```python
from build123d import *

# Parameters (mm, degrees)
PLASTINA_DEPTH        = 5
OTVERSTIYA_DEPTH      = 86
OTVERSTIYA_DEPTH_BACK = 86
ESKIZ_OTVERSTIYA_R    = 1.65
ESKIZ_OTVERSTIYA_R_2  = 11.25


with BuildPart() as part:
    # Eskiz_kontur → Plastina (new body)
    with BuildSketch(Plane.XY):
        with BuildLine():
            Line((-60, -50), (-60, 50))
            ThreePointArc((-60, 50), (-57.071067812, 57.071067812), (-50, 60))
            Line((-50, 60), (50, 60))
            ThreePointArc((50, 60), (57.071067812, 57.071067812), (60, 50))
            Line((60, 50), (60, -50))
            ThreePointArc((60, -50), (57.071067812, -57.071067812), (50, -60))
            Line((50, -60), (-50, -60))
            ThreePointArc((-50, -60), (-57.071067812, -57.071067812), (-60, -50))
        make_face()
    extrude(amount=PLASTINA_DEPTH)

    # Eskiz_otverstiya → Otverstiya (cut, two sides: drawn at the far end of the back side and taken through both)
    with BuildSketch(Plane.XY.offset(-OTVERSTIYA_DEPTH_BACK)):
        with Locations((-50, -50)):
            Circle(ESKIZ_OTVERSTIYA_R)
        with Locations((0, -36)):
            Circle(ESKIZ_OTVERSTIYA_R)
        with Locations((-15.5, -15.5)):
            Circle(ESKIZ_OTVERSTIYA_R)
        Circle(ESKIZ_OTVERSTIYA_R_2)
        with Locations((50, -50)):
            Circle(ESKIZ_OTVERSTIYA_R)
        with Locations((15.5, -15.5)):
            Circle(ESKIZ_OTVERSTIYA_R)
        with Locations((36, 0)):
            Circle(ESKIZ_OTVERSTIYA_R)
        with Locations((-36, 0)):
            Circle(ESKIZ_OTVERSTIYA_R)
        with Locations((-15.5, 15.5)):
            Circle(ESKIZ_OTVERSTIYA_R)
        with Locations((-50, 50)):
            Circle(ESKIZ_OTVERSTIYA_R)
        with Locations((0, 36)):
            Circle(ESKIZ_OTVERSTIYA_R)
        with Locations((15.5, 15.5)):
            Circle(ESKIZ_OTVERSTIYA_R)
        with Locations((50, 50)):
            Circle(ESKIZ_OTVERSTIYA_R)
    extrude(amount=OTVERSTIYA_DEPTH + OTVERSTIYA_DEPTH_BACK, mode=Mode.SUBTRACT)


solid = part.part
```
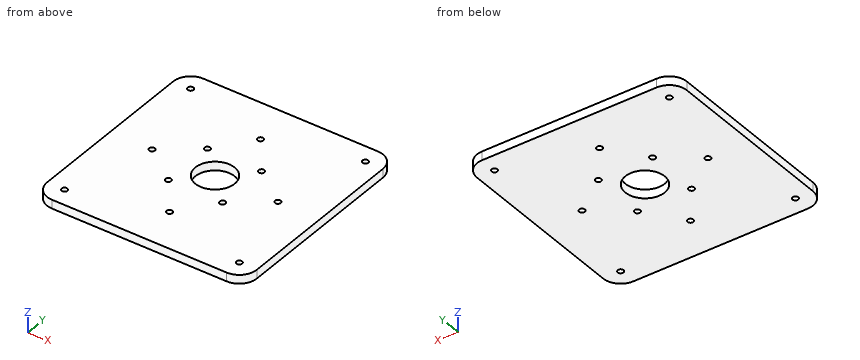
Model file for the job. Use its own axes, mm. Coordinates: 2 decimals unless noted, no trailing zeros. Loops run counter-clockwise (first coordinate to the right, second up) from the corner with the lowest first, then second, coordinate; pieces in that order, holes last. Notation, with made-up numbers: (68.25, 10.25) - (76.25, 10.25) arc R19 ccw to (76.25, 18.25) - close; hole circle Ø1 at (-20, -3). An arc over 180 degrees is marked (long way). Answer as a JSON object with one key per item and string values. Group by question number.
(1) Cut at A-A (z = 1.75). State how many separate pieces and enclosed holes the cut face has, then the cut area to 3 significant figures.
(2) Cut at B-B (x = -36). Give the cut face in (y, z).
(3) Probe line 1 along Y through (x, z) = (-50, 3.9); line 2 along Y through (x, z) = (0, 3.3); line 3 along Y through (x, z) = (15.5, 3.6). List the from-to ranges inside material, lowest first.
(4) Cut at D-D (x = 0). Give the cut face in (y, z), then the cut area to 4 significant figures.
(5) Flat gauge pins, fed straight in: pin 1 (4 mm diameter, centred on x = -46.5, y = 45, fed in from -Z); pin 2 (20 mm diameter, centred on x = 0, y = 0, fed in from +Z). Where does each tip first touch, or does it go through?
Geometry says:
{
 "1": {"separate pieces": "1", "enclosed holes": "13", "area": "13,800 mm^2"},
 "2": {"outline": "(-60, 0) - (-1.65, 0) - (-1.65, 5) - (-60, 5) - close; (1.65, 0) - (60, 0) - (60, 5) - (1.65, 5) - close"},
 "3": {"line 1": "y = -60 to -51.65, -48.35 to 48.35, 51.65 to 60", "line 2": "y = -60 to -37.65, -34.35 to -11.25, 11.25 to 34.35, 37.65 to 60", "line 3": "y = -60 to -17.15, -13.85 to 13.85, 17.15 to 60"},
 "4": {"outline": "(-60, 0) - (-37.65, 0) - (-37.65, 5) - (-60, 5) - close; (-34.35, 0) - (-11.25, 0) - (-11.25, 5) - (-34.35, 5) - close; (11.25, 0) - (34.35, 0) - (34.35, 5) - (11.25, 5) - close; (37.65, 0) - (60, 0) - (60, 5) - (37.65, 5) - close", "area": "454.5 mm^2"},
 "5": {"pin 1": "stops at z = 0", "pin 2": "passes through"}
}
